Autodesk Inventor part; units mm, degrees
ref_plane "YZ Plane" through (0, 0, 0) normal (1, 0, 0) x (0, 1, 0)
ref_plane "XZ Plane" through (0, 0, 0) normal (0, 1, 0) x (-1, 0, 0)
ref_plane "XY Plane" through (0, 0, 0) normal (0, 0, 1) x (1, 0, 0)
sketch "Sketch4" plane through (0, 0, 0) normal (0, 1, 0) x (-1, 0, 0)
  line L0 (40, -40) -> (-40, -40)
  line L1 (-40, -40) -> (-40, 0)
  line L2 (-40, 0) -> (40, 0)
  line L3 (40, 0) -> (40, -40)
  point P0 (0, 0)
  point P1 (0, 0)
  dimension "d36" = 80
  dimension "d37" = 40
extrude "Plate2" add sketch "Sketch4" along normal blind 3
sketch "Sketch5" plane through (0, 0, 0) normal (0, -1, 0) x (1, 0, 0)
  circle A0 centre (-25, -25) radius 6.5
  circle A1 centre (25, -25) radius 6.5
  line L0 (0, 0) -> (0, -40) construction
  line L1 (40, -40) -> (-40, -40) construction
  dimension "d39" = 50
  dimension "d40" = 15
  dimension "d41" = 13
extrude "Cut1" cut sketch "Sketch5" against normal blind 3
sketch "Sketch6" plane through (-40, 3, -3) normal (0, 0, 1) x (1, 0, 0)
  line L0 (80, 0) -> (0, 0)
  line L1 (0, 0) -> (0, -40)
  line L2 (0, -40) -> (80, -40)
  line L3 (80, -40) -> (80, 0)
edge flange "Flange1" height 40 angle 90 thickness 3 bend radius 5 thickness toward (0, 0, 1) relief round relief width 3 relief depth 1.5 edges at (0, 0, 0) wall of the first edge with corners at (40, 3, -3) (-40, 3, -3) (-40, -37, -3) (40, -37, -3)
bend "Bend1"
corner "Corner1"
fillet "Corner Round6" radius 6 4 edges at (40, -37, -1.5) (-40, 1.5, -40) (40, 1.5, -40) (-40, -37, -1.5)
equation "\"d42\" = Thickness"
equation "\"d38\" = Thickness"
equation "\"d44\" = BendReliefWidth"
equation "\"d45\" = BendReliefDepth"
equation "\"d46\" = MinimumRemnant"
equation "\"d47\" = TransitionRadius"
equation "\"d50\" = BendRadius"
equation "\"d51\" = CornerReliefSize"
equation "\"d52\" = GapSize"
equation "\"d53\" = JacobiRadiusSize"
equation "\"BendReliefWidth\" = Thickness"
equation "\"BendReliefDepth\" = 0.5 * Thickness"
equation "\"CornerReliefSize\" = 4 * Thickness"
equation "\"MinimumRemnant\" = 2 * Thickness"
equation "\"TransitionRadius\" = BendRadius"
equation "\"JacobiRadiusSize\" = BendRadius"
equation "\"GapSize\" = Thickness"
properties part number "MSC 912 flange slipway" material "Stainless Steel"
Check sheet for the modelled part. Datum: model origin and axes. Units: mm. A direction names the side the tool comes from. Give positions to 0.01 mm unless a question says otherwise; leave off trailing zeros. Write each loop counter-clockwise with the first axis right and the second up, starting at its lowest first coordinate (ties: lowest second). Pieces come first, ordered by that corner, then holes.
Item 1: Cross-section at A-A (x = 26.5). Enter the section's corners in (y, z), and give its area (3 significant figures).
Item 2: Gauge pin test, flat ends, axial feed: pin 1 (12 mm diameter, centred on x = -17, y = -15.5, fed in from -Z); pin 2 (2 mm diameter, centred on x = -21, z = -20.5, fed in from -Y); pin 3 (10 mm diameter, centred on y = -21, z = -10.5, fed in from -X). Record the tip position at first contact, or that the pin passes through.
Item 3: Draft check along X on faces 1 (the face through (20.209, 1.479, -20.607)), 2 (the face through (0, 1, -40)), 3 (the face through (40, -1, -4)). Enter one of: released by +X, released by -X, zero draft, split by the parting line, or undercut.
Item 4: Access from +Z, -Z, +X, -X, +Y, -Y to the whole of each face (thin tool, end or side, straight path). Record for faces 4 (the face through (-0.56, 0.594, -2.281)), 5 (the face through (1, 0, -24)).
Item 5: Scan lines: L1, parallel to Y at x = -33, z = -9; L2, parallel to Z at x = 25, y = 2.3; L3, parallel to Z at x = -25, y = 1. Record each from-to range of solid material in increasing order.
Item 6: Cross-section at D-D (x = -25). Enter the section's corners in (y, z).
Item 7: Cross-section at C-C (x = -3). Enter the section's corners in (y, z).
Item 8: Cross-section at B-B (z = -25). Enter the section's corners in (x, y).
Report:
1. outline: (-37, -3) - (-5, -3) arc R5 cw to (0, -8) - (0, -18.68) - (3, -18.68) - (3, -8) arc R8 ccw to (-5, 0) - (-37, 0) - close; (0, -40) - (3, -40) - (3, -31.32) - (0, -31.32) - close
1. area: 185 mm2
2. pin 1: stops at z = -3
2. pin 2: stops at y = 0
2. pin 3: passes through
3. face 1: undercut
3. face 2: zero draft
3. face 3: released by +X
4. face 4: +Z, +X, -X, +Y
4. face 5: -Z, +X, -X, -Y
5. L1: y = 0 to 3
5. L2: z = -40 to -31.5, -18.5 to -4.73
5. L3: z = -40 to -31.5, -18.5 to -2.71
6. outline: (-37, -3) - (-5, -3) arc R5 cw to (0, -8) - (0, -18.5) - (3, -18.5) - (3, -8) arc R8 ccw to (-5, 0) - (-37, 0) - close; (0, -40) - (3, -40) - (3, -31.5) - (0, -31.5) - close
7. outline: (-37, -3) - (-5, -3) arc R5 cw to (0, -8) - (0, -40) - (3, -40) - (3, -8) arc R8 ccw to (-5, 0) - (-37, 0) - close
8. outline: (-40, 0) - (-31.5, 0) - (-31.5, 3) - (-40, 3) - close; (-18.5, 0) - (18.5, 0) - (18.5, 3) - (-18.5, 3) - close; (31.5, 0) - (40, 0) - (40, 3) - (31.5, 3) - close
